Work out the finished part from the listing and answer in its coordinate system (mm). A direction names the side the tool comes from. Round coordinates to 2 decimals unless told otherwise and drop trailing zeros. Order: outer loops, then holes, each group sorted by start corner. A loop starts at its lowest first (then second) coordinate and runs counter-clockwise, first axis right, second up. Notation, with made-up numbers: (-22.5, 89) -> (-10.5, 89) arc R19 ccw to (-10.5, 115) -> close; hole circle Ø9 at (46, -16.5). An arc over 180 degrees is marked (long way). Use one line per item in the form item = value.
```python
from build123d import *

# Parameters (mm, degrees)
F2_R     = 0.057539
F3_DEPTH = 12.7
F4_R     = 3.113486
F5_DEPTH = 1.524
F6_R     = 1.696249
F7_DEPTH = 27.432


with BuildPart() as f1:
    # F0 (on Front) → F1 (revolve)
    with BuildSketch(Plane.XZ):
        Polygon((-2.54, 0), (0, 0), (0, 12.033645), (-5.08, 12.033645), align=None)
    revolve(axis=Axis((0, 0, 6.016822), (0, 0, -1)))

    # F2 (on Right) → F3 (cut, symmetric)
    with BuildSketch(Plane.YZ):
        with Locations((0, 19.658387)):
            Circle(F2_R)
    extrude(amount=F3_DEPTH, both=True, mode=Mode.SUBTRACT)

    # F4 (on Front) → F5 (join)
    with BuildSketch(Plane.XZ):
        with Locations((0, 13.446124)):
            Circle(F4_R)
    extrude(amount=F5_DEPTH)

    # F6 (on Front) → F7 (cut)
    with BuildSketch(Plane.XZ):
        with Locations((0, 13.890625)):
            Circle(F6_R)
    extrude(amount=F7_DEPTH, mode=Mode.SUBTRACT)


solid = f1.part
```
Item 1: For faces 1 (the flat face through (0, -1.524, 16)), 2 (the flat face through (0, 0, 0)), determine the directions among +Z, -Z, +X, -X, +Y, -Y from which every point of the face is accessible in a straight line to the end or side of a thin tool.
Findings:
face_1 = +Z, +X, -X, -Y
face_2 = -Z, +X, -X, +Y, -Y
Item 2: Determine the mould class of faces 3 (the conical face through (-3.35, 1.05, 4.6)), 4 (the flat face through (0, 0, 16)), 5 (the cylindrical face through (1.62, -0.75, 14.4)) for opening direction X: released by +X, released by -X, zero draft, split by the parting line, or undercut.
Findings:
face_3 = split by the parting line
face_4 = zero draft
face_5 = undercut
Item 3: Consider line 1 along Z through (x, y) = (0, -0.55); line 2 along Z through (x, y) = (-0.5, 2.25); line 3 along Y through (x, z) = (-2.75, 14.25). Determine where each line is inside the solid, lowest interval first.
Findings:
line_1 = 0 to 12.19, 15.59 to 16.56
line_2 = 0 to 12.03
line_3 = -1.52 to 0
Item 4: The part is cut by section B-B, the plane z = 8.25. Give the vertices of the cut face in (x, y), and give its area (3 significant figures).
Findings:
outline = circle Ø8.56 at (0, 0)
area = 57.6 mm^2
Item 5: The part is cut by section C-C, the plane z = 4. Give the vertices of the cut face in (x, y).
Findings:
outline = circle Ø6.77 at (0, 0)
Item 6: Flat-ended cylindrical pins translate along their axes: P1, Ø2, axis at x = 1, z = 12.5, coming from the -Y side; P2, Ø2.5, axis at x = -1.5, z = 14, coming from the -Y side; P3, Ø4, axis at y = -3, z = 2, coming from the -X side. Find the tip coordinate at first contact, or state that the pin passes through.
Findings:
P1 = -5.08
P2 = -1.52
P3 = -2.91
Item 7: The part is cut by section A-A, the plane x = 0. Give the vertices of the cut face in (y, z).
Findings:
outline = (-5.08, 12.03) -> (-2.54, 0) -> (2.54, 0) -> (5.08, 12.03) -> (0, 12.03) -> (0, 12.19) -> (-1.52, 12.19) -> (-1.52, 12.03) -> close; (-1.52, 15.59) -> (0, 15.59) -> (0, 16.56) -> (-1.52, 16.56) -> close
